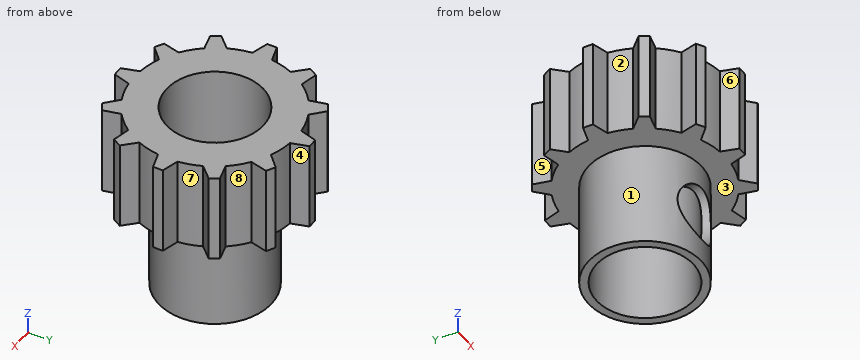
from build123d import *

# Parameters (mm, degrees)
SKETCH1_R           = 5
SKETCH1_R_2         = 3
BOSS_EXTRUDE1_DEPTH = 5.5
BOSS_EXTRUDE2_START = -5.5
BOSS_EXTRUDE2_DEPTH = 5.5
CIRPATTERN1_COUNT   = 12
BOSS_EXTRUDE3_START = -6.5
SKETCH4_R           = 3.5
SKETCH4_R_2         = 3
BOSS_EXTRUDE3_DEPTH = 6.5
SKETCH5_R           = 1.75
CUT_EXTRUDE1_DEPTH  = 6.5


with BuildPart() as part:
    # Sketch1 → Boss-Extrude1 (new body)
    with BuildSketch(Plane.XY):
        Circle(SKETCH1_R)
        Circle(SKETCH1_R_2, mode=Mode.SUBTRACT)
    extrude(amount=BOSS_EXTRUDE1_DEPTH)

    # Sketch3 → Boss-Extrude2 (add)
    with BuildSketch(Plane.XY.offset(5.5).offset(BOSS_EXTRUDE2_START)):
        with BuildLine():
            Line((-0.3, -5.992495307), (-0.6, -4.963869458))
            ThreePointArc((-0.6, -4.963869458), (0, -5), (0.6, -4.963869458))
            Line((0.6, -4.963869458), (0.3, -5.992495307))
            ThreePointArc((0.3, -5.992495307), (0, -6), (-0.3, -5.992495307))
        make_face()
    boss_extrude2 = extrude(amount=BOSS_EXTRUDE2_DEPTH)

    # CirPattern1: Boss-Extrude2 ×12 about axis
    cirpattern1_axis = Axis((0, 0, 0), (0, 0, 1))
    for i in range(1, CIRPATTERN1_COUNT):
        add(boss_extrude2.rotate(cirpattern1_axis, i * 360 / CIRPATTERN1_COUNT))

    # Sketch4 → Boss-Extrude3 (add)
    with BuildSketch(Plane.XY.offset(BOSS_EXTRUDE3_START)):
        Circle(SKETCH4_R)
        Circle(SKETCH4_R_2, mode=Mode.SUBTRACT)
    extrude(amount=BOSS_EXTRUDE3_DEPTH)

    # Sketch5 → Cut-Extrude1 (cut)
    with BuildSketch(Plane(origin=(0, 0, 0), x_dir=(1, 0, 0), z_dir=(0, 1, 0))):
        with Locations(Location((0, 3.25, 0), (0, 0, 270))):
            Circle(SKETCH5_R)
    extrude(amount=-CUT_EXTRUDE1_DEPTH, mode=Mode.SUBTRACT)


solid = part.part
Check sheet for the modelled part. Datum: model origin and axes. Units: mm. Face numbers are marked on the shaded views. A direction names the side the tool comes from. Give positions to 0.01 mm unless a question says otherwise; leave off trailing zeros. Loops run counter-clockwise (first coordinate to the right, second up) from the corner with the lowest first, then second, coordinate; pieces in that order, holes last. Notation, with made-up numbers: M 16,81.25 L 74,81.25 A19 ccw 74,96.25 Z; hole C 52,-2 d5. An arc over 180 degrees is marked long. Return JSON: item names as keys, results as strings. Group by question number.
1. Go/stop test with flat-tipped pins: pin 1 (1.5 mm diameter, centred on y = -2.5, z = -2, fed in from +X); pin 2 (2 mm diameter, centred on x = 4, y = 2.5, fed in from -Z); pin 3 (1.5 mm diameter, centred on x = -2.5, z = 3, fed in from -Y); pin 4 (3.5 mm diameter, centred on x = 0, y = 0, fed in from +Z). Record where each tip stops, or that it passes through.
2. Thickness scan on L1, parallel to Y at x = 0, z = -0.5; L2, parallel to X at y = -5, z = 2.5; L3, parallel to X at y = -2.9, z = -3.25. Record the ranges inside material, lowest first.
3. Cross-section at C-C on y = -1.75. Record the boundary of the cut face in (x, z).
4. Cross-section at A-A on x = 0. Record the boundary of the cut face in (y, z), plus the area to 4 significant figures.
5. Cross-section at B-B on y = 0. Record the boundary of the cut face in (x, z), plus the area to 3 significant figures.
6. Cross-section at D-D on z = -3.25. Record the boundary of the cut face in (x, y).
7. Tool access check on the marked faces 4, 5, 6, 7 and 8. Record the directions out of +Z, -Z, +X, -X, +Y, -Y that give a thin tool (end or side, any length) a straight path to the whole face; none if there is none.
8. Mould release check, pull along Y, two halves, no side actions. Record for the marked faces 1, 2 and 3: released by +Y, released by -Y, zero draft, split by the parting line, or undercut.
Return value:
{
 "1": {"pin 1": "x = 3.03", "pin 2": "z = 0", "pin 3": "y = -5.34", "pin 4": "through"},
 "2": {"L1": "-3.5 to -3, 3 to 3.5", "L2": "-3.25 to -2.38, -0.59 to 0.59, 2.38 to 3.25", "L3": "-1.96 to -1.75, 1.75 to 1.96"},
 "3": {"outline": "M -4.68,0 L -3.03,0 L -3.03,-6.5 L -2.44,-6.5 L -2.44,5.5 L -4.68,5.5 Z; M 2.44,-6.5 L 3.03,-6.5 L 3.03,0 L 4.68,0 L 4.68,5.5 L 2.44,5.5 Z"},
 "4": {"outline": "M -6,0 L -3.5,0 L -3.5,-1.5 L -3,-1.5 L -3,5.5 L -6,5.5 Z; M -3.5,-6.5 L -3,-6.5 L -3,-5 L -3.5,-5 Z; M 3,-6.5 L 3.5,-6.5 L 3.5,0 L 6,0 L 6,5.5 L 3,5.5 Z", "area": "37.75 mm^2"},
 "5": {"outline": "M -6,0 L -3.5,0 L -3.5,-6.5 L -3,-6.5 L -3,5.5 L -6,5.5 Z; M 3,-6.5 L 3.5,-6.5 L 3.5,0 L 6,0 L 6,5.5 L 3,5.5 Z", "area": "39.5 mm^2"},
 "6": {"outline": "M -1.75,-3.03 L -1.75,-2.44 A3 cw long 1.75,-2.44 L 1.75,-3.03 A3.5 ccw long Z"},
 "7": {"face 4": "+Z, -Z, +Y", "face 5": "+Z, -Z, -X", "face 6": "+Z, -Z, -Y", "face 7": "+Z, -Z, +X", "face 8": "+Z, -Z"},
 "8": {"face 1": "split by the parting line", "face 2": "undercut", "face 3": "zero draft"}
}
